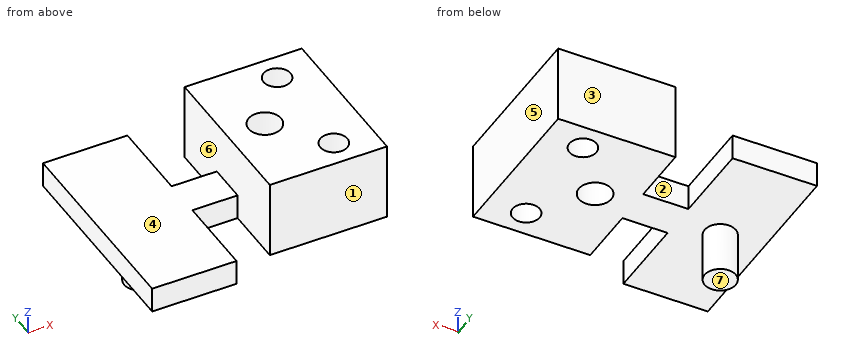
Autodesk Inventor part; units mm, degrees
ref_plane "YZ Plane" through (0, 0, 0) normal (1, 0, 0) x (0, 1, 0)
ref_plane "XZ Plane" through (0, 0, 0) normal (0, 1, 0) x (-1, 0, 0)
ref_plane "XY Plane" through (0, 0, 0) normal (0, 0, 1) x (1, 0, 0)
sketch "Skizze1" plane through (0, 0, 0) normal (0, 0, 1) x (1, 0, 0)
  circle A0 centre (-2.545, 0) radius 7.475
  circle A1 centre (-2.545, 0) radius 1.5
  circle A2 centre (1.205, -4.91) radius 1.25
  circle A3 centre (1.205, 4.91) radius 1.25
  line L0 (-6.025, -7.365) -> (4.805, -7.365)
  line L1 (4.805, -7.365) -> (4.805, 7.365)
  line L2 (4.805, 7.365) -> (-6.025, 7.365)
  line L3 (-6.025, 7.365) -> (-6.025, -7.365)
  line L4 (-6.025, -7.365) -> (4.805, 7.365) construction
  line L5 (4.805, -7.365) -> (-6.025, 7.365) construction
  line L6 (-10.205, -1.8) -> (-6.025, -1.8)
  line L7 (-6.025, -1.8) -> (-6.025, 1.8)
  line L8 (-6.025, 1.8) -> (-10.205, 1.8)
  line L9 (-10.205, 1.8) -> (-10.205, -1.8)
  line L10 (-10.205, -1.8) -> (-6.025, 1.8) construction
  line L11 (-6.025, -1.8) -> (-10.205, 1.8) construction
  line L12 (-18.005, -9.44) -> (-10.205, -9.44)
  line L13 (-10.205, -9.44) -> (-10.205, 9.44)
  line L14 (-10.205, 9.44) -> (-18.005, 9.44)
  line L15 (-18.005, 9.44) -> (-18.005, -9.44)
  line L16 (-18.005, -9.44) -> (-10.205, 9.44) construction
  line L17 (-10.205, -9.44) -> (-18.005, 9.44) construction
  point P0 (0, 0)
  point P1 (-0.61, 0)
  point P2 (-8.115, 0)
  point P3 (-6.025, 0)
  point P4 (-14.105, 0)
  point P5 (-10.205, 0)
  dimension "d1" = 3.6
  dimension "d2" = 14.73
  dimension "d3" = 10.83
  dimension "d4" = 4.18
  dimension "d5" = 3.6
  dimension "d6" = 18.88
  dimension "d7" = 7.8
extrude "Extrusion1" add sketch "Skizze1" along normal blind 2.35 contours L1 A0 L0 L3 L2 | A0 L2 L1 | L1 L0 A0 | A0 L3 L2 | L0 L3 A0 | L8 L3 L6 A0 | A0 L6 L9 L8 | L9 L13 L12 L15 L14
sketch "Skizze2" plane through (0, 0, 2.35) normal (0, 0, 1) x (1, 0, 0)
  line L0 (-10.205, -9.44) -> (-10.205, -1.8)
  line L1 (-10.205, -1.8) -> (-6.025, -1.8)
  line L2 (-6.025, -1.8) -> (-6.025, -7.365)
  line L3 (-6.025, -7.365) -> (4.805, -7.365)
  line L4 (4.805, -7.365) -> (4.805, 7.365)
  line L5 (4.805, 7.365) -> (-6.025, 7.365)
  line L6 (-6.025, 7.365) -> (-6.025, 1.8)
  line L7 (-6.025, 1.8) -> (-10.205, 1.8)
  line L8 (-10.205, 1.8) -> (-10.205, 9.44)
  line L9 (-10.205, 9.44) -> (-18.005, 9.44)
  line L10 (-18.005, 9.44) -> (-18.005, -9.44)
  line L11 (-18.005, -9.44) -> (-10.205, -9.44)
  circle A0 centre (1.205, 4.91) radius 1.25
  circle A1 centre (1.205, -4.91) radius 1.25
  circle A2 centre (-2.545, 0) radius 1.5
  line L12 (-6.025, 1.8) -> (-10.205, 1.8)
  line L13 (-6.025, 1.8) -> (-6.025, -1.8)
  point P0 (0, 0)
extrude "Extrusion2" add sketch "Skizze2" along normal blind 4.9 contours L13 L6 L5 L4 L3 L2
sketch "Skizze3" plane through (0, 0, 0) normal (0, 0, -1) x (-1, 0, 0)
  line L0 (10.205, -9.44) -> (10.205, -1.8)
  line L1 (18.005, -9.44) -> (10.205, -9.44)
  line L2 (18.005, 9.44) -> (18.005, -9.44)
  line L3 (10.205, 9.44) -> (18.005, 9.44)
  line L4 (10.205, 1.8) -> (10.205, 9.44)
  line L5 (6.025, 1.8) -> (10.205, 1.8)
  line L6 (6.025, 7.365) -> (6.025, 1.8)
  line L7 (-4.805, 7.365) -> (6.025, 7.365)
  line L8 (-4.805, -7.365) -> (-4.805, 7.365)
  line L9 (6.025, -7.365) -> (-4.805, -7.365)
  line L10 (6.025, -1.8) -> (6.025, -7.365)
  line L11 (10.205, -1.8) -> (6.025, -1.8)
  circle A0 centre (-1.205, 4.91) radius 1.25
  circle A1 centre (-1.205, -4.91) radius 1.25
  circle A2 centre (2.545, 0) radius 1.5
  circle A3 centre (14.105, 0) radius 1.435
  point P0 (0, 0)
  dimension "d12" = 2.87
extrude "Extrusion3" add sketch "Skizze3" along normal blind 4.64 contours A3
properties part number "00_Linear_Stepper_90mm_slide"
Geometry check sheet. Reference: the model listing, model coordinates, mm. Face numbers are marked on the shaded views. A direction names the side the tool comes from. Give positions to 0.01 mm unless a question says otherwise; leave off trailing zeros. Order: outer loops, then holes, each group sorted by start corner. A loop starts at its lowest first (then second) coordinate and runs counter-clockwise, first axis right, second up.
1. Section check D-D, the plane y = 2.25. Enter the section's corners in (x, z) (3 decimals).
2. Gauge pin test, flat ends, axial feed: pin 1 Ø0.7 at (x, z) = (-9, 1) entering from +Y; pin 2 Ø2 at (y, z) = (1.5, 3.5) entering from -X (3 decimals); pin 3 Ø3 at (x, y) = (1, 5.5) entering from -Z. Record the tip position at first contact, or that the pin passes through.
3. Section check B-B, the plane z = 6. Enter the section's corners in (x, y) (3 decimals), and give its area (3 significant figures).
4. Thickness scan on L1, parallel to X at y = 6.75, z = 1.75 (3 decimals); L2, parallel to Z at x = -14, y = -7; L3, parallel to X at y = 5, z = 3 (3 decimals). Record the ranges inside material, lowest first.
5. Access from +Z, -Z, +X, -X, +Y, -Y to the whole of each face (thin tool, end or side, straight path). Record for the marked faces 1, 2, 3 and 4.
6. Section check C-C, the plane y = 4.91. Enter the section's corners in (x, z) (3 decimals), and give its area (3 significant figures).
7. Release check for a two-part mould opening along X. For the marked faces 5, 6 and 7 record: pulls with the +X half, pulls with the -X half, needs draft (parallel to the pull), parting line crosses it, or undercut.
8. Section check A-A, the plane y = 0. Enter the section's corners in (x, z) (3 decimals).
Values follow:
1. outline: (-18.005, 0) - (-10.205, 0) - (-10.205, 2.35) - (-18.005, 2.35) - close; (-6.025, 0) - (4.805, 0) - (4.805, 7.25) - (-6.025, 7.25) - close
2. pin 1: stops at y = 1.8
2. pin 2: stops at x = -6.025
2. pin 3: stops at z = 0
3. outline: (-6.025, -7.365) - (4.805, -7.365) - (4.805, 7.365) - (-6.025, 7.365) - close; hole circle Ø3 at (-2.545, 0); hole circle Ø2.5 at (1.205, -4.91); hole circle Ø2.5 at (1.205, 4.91)
3. area: 143 mm2
4. L1: x = -18.005 to -10.205, -6.025 to 4.805
4. L2: z = 0 to 2.35
4. L3: x = -6.025 to -0.042, 2.452 to 4.805
5. face 1: +Z, -Z, +X, -Y
5. face 2: +Z, -Z, +Y
5. face 3: +Z, -Z, +X, +Y
5. face 4: +Z, -X, +Y, -Y
6. outline: (-18.005, 0) - (-10.205, 0) - (-10.205, 2.35) - (-18.005, 2.35) - close; (-6.025, 0) - (-0.045, 0) - (-0.045, 7.25) - (-6.025, 7.25) - close; (2.455, 0) - (4.805, 0) - (4.805, 7.25) - (2.455, 7.25) - close
6. area: 78.7 mm2
7. face 5: pulls with the +X half
7. face 6: undercut
7. face 7: needs draft
8. outline: (-18.005, 0) - (-15.54, 0) - (-15.54, -4.64) - (-12.67, -4.64) - (-12.67, 0) - (-4.045, 0) - (-4.045, 7.25) - (-6.025, 7.25) - (-6.025, 2.35) - (-18.005, 2.35) - close; (-1.045, 0) - (4.805, 0) - (4.805, 7.25) - (-1.045, 7.25) - close
